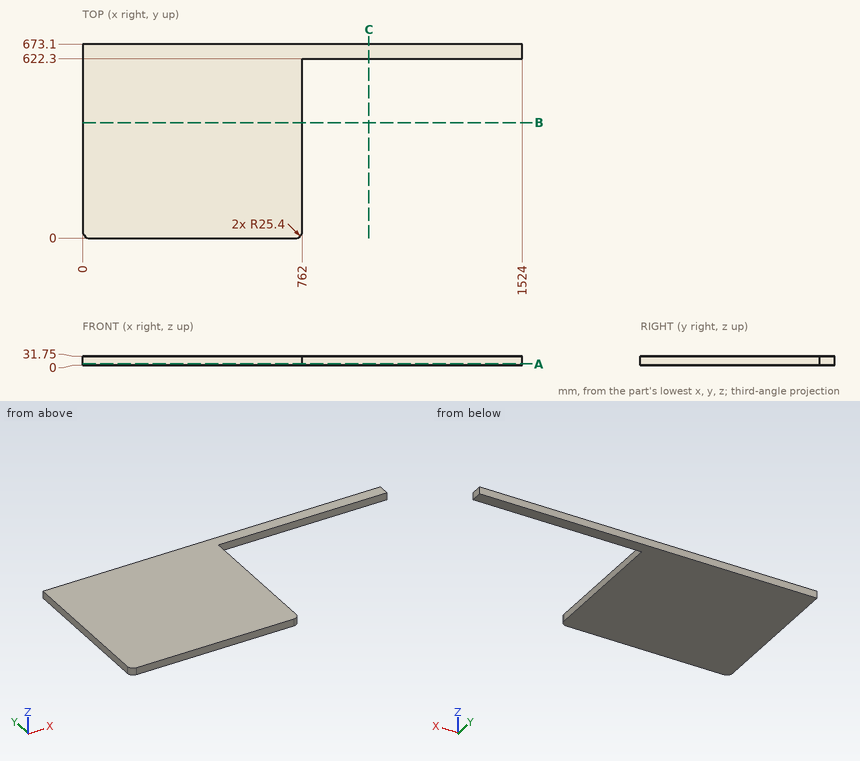
Could you check a few things on this drawing? It's one solid part, dimensions in mm from its lowest x, y, z. Give positions to 0.01 mm unless a question says otherwise; leave off trailing zeros. Order: outer loops, then holes, each group sorted by start corner. A loop starts at its lowest first (then second) coordinate and runs counter-clockwise, first axis right, second up. Notation, with made-up numbers: (10, -19) - (44, -19) arc R26 cw to (44, -3) - close; hole circle Ø4 at (71.5, -8). An arc over 180 degrees is marked (long way). One line per item, written item: value. Start each with the question number.
1. If I drill on probe 1 along X at (y, z) = (63, 9); probe 2 along Y at (x, z) = (1278, 6.5); probe 3 along Y at (x, z) = (748, 20), over which ranges is the centre line in solid material (lowest first)?
2. Imagine slicing it at C-C on x = 992.5. List the corners of the cut face in (y, z) for me, plus the area to 3 significant figures.
3. Imagine slicing it at A-A on z = 5.5. List the corners of the cut face in (x, y) for me, plus the area to 3 significant figures.
4. For P1, Ø9.5, axis at y = 177, z = 21, coming from the +X side, with a flat end and sliding along its axis, tell me the tip position at first contact or that it passes through.
5. Imagine slicing it at B-B on y = 400.5. List the corners of the cut face in (x, z) for me.
Values:
1. probe 1: 0 to 762
1. probe 2: 622.3 to 673.1
1. probe 3: 2.7 to 673.1
2. outline: (622.3, 0) - (673.1, 0) - (673.1, 31.75) - (622.3, 31.75) - close
2. area: 1,610 mm²
3. outline: (0, 25.4) arc R25.4 ccw to (25.4, 0) - (736.6, 0) arc R25.4 ccw to (762, 25.4) - (762, 622.3) - (1524, 622.3) - (1524, 673.1) - (0, 673.1) - close
3. area: 551,000 mm²
4. P1: x = 762
5. outline: (0, 0) - (762, 0) - (762, 31.75) - (0, 31.75) - close
